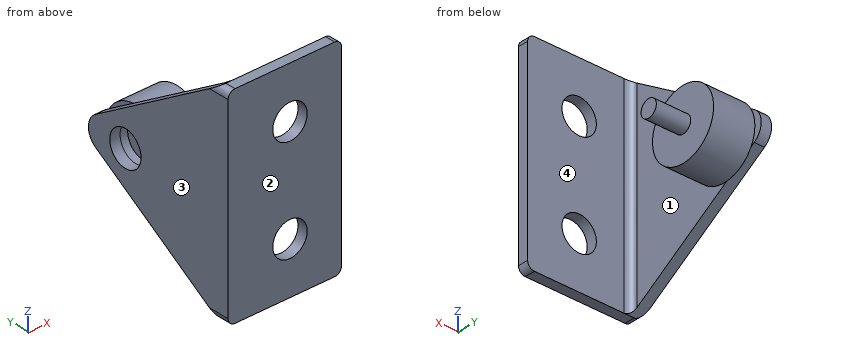
from build123d import *

# Parameters (mm, degrees)
BOSS_EXTRUDE1_DEPTH = 38.1
CUT_EXTRUDE2_DEPTH  = 76.2
FILLET1_R           = 6.35
SKETCH10_W          = 21.59
SKETCH10_H          = 76.2
CUT_EXTRUDE3_DEPTH  = 76.2
FILLET2_R           = 2.54
FILLET3_R           = 2.54
SKETCH11_R          = 6.5024
CUT_EXTRUDE4_DEPTH  = 76.2
SKETCH12_R          = 6.35
CUT_EXTRUDE5_DEPTH  = 76.2
SKETCH13_R          = 12.7
BOSS_EXTRUDE2_DEPTH = 15.24
CUT_EXTRUDE6_START  = -6.604
SKETCH17_R          = 6.5024
CUT_EXTRUDE6_DEPTH  = 6.604
SKETCH18_R          = 3.175
BOSS_EXTRUDE3_DEPTH = 12.7


with BuildPart() as part:
    # Sketch7 → Boss-Extrude1 (new, symmetric)
    with BuildSketch(Plane.XY):
        Polygon((0, 0), (0, 63.5), (3.81, 63.5), (3.81, 3.81), (63.5, 3.81), (63.5, 0), align=None)
    extrude(amount=BOSS_EXTRUDE1_DEPTH, both=True)

    # Sketch8 → Cut-Extrude2 (cut)
    with BuildSketch(Plane(origin=(3.81, 0, 0), x_dir=(0, 0, -1), z_dir=(1, 0, 0))):
        Polygon((-38.1, 63.5), (-38.1, 3.81), (0, 63.5), align=None)
        Polygon((38.1, 63.5), (0, 63.5), (38.1, 3.81), align=None)
    extrude(amount=-CUT_EXTRUDE2_DEPTH, mode=Mode.SUBTRACT)

    # Fillet1
    fillet1_edges = [part.edges().sort_by_distance(p)[0] for p in [
        (1.905, 63.5, 0),
    ]]
    fillet(fillet1_edges, radius=FILLET1_R)

    # Sketch10 → Cut-Extrude3 (cut)
    with BuildSketch(Plane(origin=(0, 3.81, 0), x_dir=(1, 0, 0), z_dir=(0, 1, 0))):
        with Locations((52.705, 0)):
            Rectangle(SKETCH10_W, SKETCH10_H)
    extrude(amount=-CUT_EXTRUDE3_DEPTH, mode=Mode.SUBTRACT)

    # Fillet2
    fillet2_edges = [part.edges().sort_by_distance(p)[0] for p in [
        (0, 1.905, 38.1),
        (0, 1.905, -38.1),
        (41.91, 1.905, -38.1),
        (41.91, 1.905, 38.1),
    ]]
    fillet(fillet2_edges, radius=FILLET2_R)

    # Fillet3
    fillet3_edges = [part.edges().sort_by_distance(p)[0] for p in [
        (3.81, 3.81, 0),
    ]]
    fillet(fillet3_edges, radius=FILLET3_R)

    # Sketch11 → Cut-Extrude4 (cut)
    with BuildSketch(Plane(origin=(3.81, 0, 0), x_dir=(0, 0, -1), z_dir=(1, 0, 0))):
        with Locations((0, 42.692021475)):
            Circle(SKETCH11_R)
    extrude(amount=-CUT_EXTRUDE4_DEPTH, mode=Mode.SUBTRACT)

    # Sketch12 → Cut-Extrude5 (cut)
    with BuildSketch(Plane(origin=(0, 3.81, 0), x_dir=(1, 0, 0), z_dir=(0, 1, 0))):
        with Locations(Location((22.86, 19.05, 0), (0, 0, 180))):
            Circle(SKETCH12_R)
        with Locations(Location((22.86, -19.05, 0), (0, 0, 180))):
            Circle(SKETCH12_R)
    extrude(amount=-CUT_EXTRUDE5_DEPTH, mode=Mode.SUBTRACT)

    # Sketch13 → Boss-Extrude2 (add)
    with BuildSketch(Plane(origin=(3.81, 0, 0), x_dir=(0, 0, -1), z_dir=(1, 0, 0))):
        with Locations(Location((0, 42.692021475, 0), (0, 0, 175.622523878))):
            Circle(SKETCH13_R)
    extrude(amount=BOSS_EXTRUDE2_DEPTH)

    # Sketch17 → Cut-Extrude6 (cut)
    with BuildSketch(Plane.ZY.offset(CUT_EXTRUDE6_START)):
        with Locations(Location((0, 42.692021475, 0), (0, 0, 180))):
            Circle(SKETCH17_R)
    extrude(amount=CUT_EXTRUDE6_DEPTH, mode=Mode.SUBTRACT)

    # Sketch18 → Boss-Extrude3 (add)
    with BuildSketch(Plane(origin=(19.05, 0, 0), x_dir=(0, 0, -1), z_dir=(1, 0, 0))):
        with Locations((0, 42.692021475)):
            Circle(SKETCH18_R)
    extrude(amount=BOSS_EXTRUDE3_DEPTH)


solid = part.part
Work out the finished part from the listing and answer in its coordinate system (mm). Face numbers are marked on the shaded views. Give positions to 0.01 mm unless a question says otherwise; leave off trailing zeros. Loops run counter-clockwise (first coordinate to the right, second up) from the corner with the lowest first, then second, coordinate; pieces in that order, holes last. Notation, with made-up numbers: (39, 40) -> (54, 40) arc R27 ccw to (54, 78) -> close; hole circle Ø6 at (17, -7.5). An arc over 180 degrees is marked (long way). Use a Markdown table: item, result. Add a question column.
1. Section C-C on x = 22.86 is taken. Determine the outline of the cut face in (y, z) (3 decimals), and give its area (3 significant figures).
2. Section D-D on z = 0 is taken. Determine the outline of the cut face in (x, y), and give its area (3 significant figures).
3. Section A-A on x = 11 is taken. Determine the outline of the cut face in (y, z), and give its area (3 significant figures).
4. Find the intervals of material crossed by probe 1 along Y at (x, z) = (2, 0); probe 2 along Z at (x, y) = (26.5, 2); probe 3 along Y at (x, z) = (6, 4), in increasing order.
5. Flat-ended cylindrical pins translate along their axes: pin 1 Ø18.5 at (y, z) = (24, -16) entering from +X; pin 2 Ø10.5 at (x, z) = (32.5, -11) entering from +Y; pin 3 Ø3.5 at (y, z) = (56, 1.5) entering from +X. Find the tip coordinate at first contact, or state that the pin passes through.
6. Section B-B on z = 19.05 is taken. Determine the outline of the cut face in (x, y) (3 decimals).
7. Determine the mould class of the marked faces 1, 2, 3 and 4 for opening direction Y: released by +Y, released by -Y, zero draft, split by the parting line, or undercut.
Results below:
| question | item | result |
|---|---|---|
| 1 | outline | (0, -38.1) -> (3.81, -38.1) -> (3.81, -25.4) -> (0, -25.4) -> close; (0, -12.7) -> (3.81, -12.7) -> (3.81, 12.7) -> (0, 12.7) -> close; (0, 25.4) -> (3.81, 25.4) -> (3.81, 38.1) -> (0, 38.1) -> close; circle Ø6.35 at (42.692, 0) |
| 1 | area | 225 mm^2 |
| 2 | outline | (0, 0) -> (41.91, 0) -> (41.91, 3.81) -> (6.35, 3.81) arc R2.54 cw to (3.81, 6.35) -> (3.81, 29.99) -> (19.05, 29.99) -> (19.05, 39.52) -> (31.75, 39.52) -> (31.75, 45.87) -> (19.05, 45.87) -> (19.05, 55.39) -> (3.81, 55.39) -> (3.81, 58.05) -> (0, 58.05) -> (0, 49.19) -> (6.6, 49.19) -> (6.6, 36.19) -> (0, 36.19) -> close |
| 2 | area | 750 mm^2 |
| 3 | outline | (0, -38.1) -> (3.81, -38.1) -> (3.81, 38.1) -> (0, 38.1) -> close; circle Ø25.4 at (42.69, 0) |
| 3 | area | 797 mm^2 |
| 4 | probe 1 | y = 0 to 36.19, 49.19 to 58.05 |
| 4 | probe 2 | z = -38.1 to -24.25, -13.85 to 13.85, 24.25 to 38.1 |
| 4 | probe 3 | y = 0 to 3.83, 30.64 to 37.57, 47.82 to 54.75 |
| 5 | pin 1 | stops at x = 3.81 |
| 5 | pin 2 | stops at y = 3.81 |
| 5 | pin 3 | stops at x = 19.05 |
| 6 | outline | (0, 0) -> (16.51, 0) -> (16.51, 3.81) -> (6.35, 3.81) arc R2.54 cw to (3.81, 6.35) -> (3.81, 33.655) -> (0, 33.655) -> close; (29.21, 0) -> (41.91, 0) -> (41.91, 3.81) -> (29.21, 3.81) -> close |
| 7 | face 1 | undercut |
| 7 | face 2 | released by -Y |
| 7 | face 3 | zero draft |
| 7 | face 4 | undercut |
